For this review, take the finished solid that the model builds, in its own axes (mm). Face numbers are marked on the shaded views. Give positions to 0.01 mm unless a question says otherwise; leave off trailing zeros. Order: outer loops, then holes, each group sorted by start corner. A loop starts at its lowest first (then second) coordinate and runs counter-clockwise, first axis right, second up.
Item 1: Consider section D-D (z = -3). Give the boundary of the cut face in (x, y), plus the area to 3 significant figures.
Item 2: Consider section C-C (y = 0.25). Give the number of separate pieces and of enclosed holes in the cut face, plus the area to 3 significant figures.
Item 3: Consider section B-B (y = 2). Give the boundary of the cut face in (x, z), plus the area to 3 significant figures.
Item 4: For probe 1 along Z at (x, y) = (-0.5, 2.7); probe 2 along Y at (x, z) = (0, -4.25), list the stretches that pass through material, from the lowest coordinate up.
Item 5: Consider section A-A (x = 0). Give the boundary of the cut face in (y, z).
Item 6: The part is to be moulded in two halves that separate along Z. For the marked faces 1, 2 and 3, say which applies: released by +Z, released by -Z, zero draft, split by the parting line, or undercut.
Item 7: For P1, Ø1, axis at x = 11, y = -2.5, coming from the +Z side; P2, Ø1.6, axis at x = 9, y = 0.5, coming from the +Z side; P3, Ø0.6, axis at x = 8, z = -1, coming from the +Y side; P4, Ø6, axis at x = 7.5, z = -1.5, coming from the -Y side, all flat-tipped, find the tip position at first contact; note any pin that passes through.
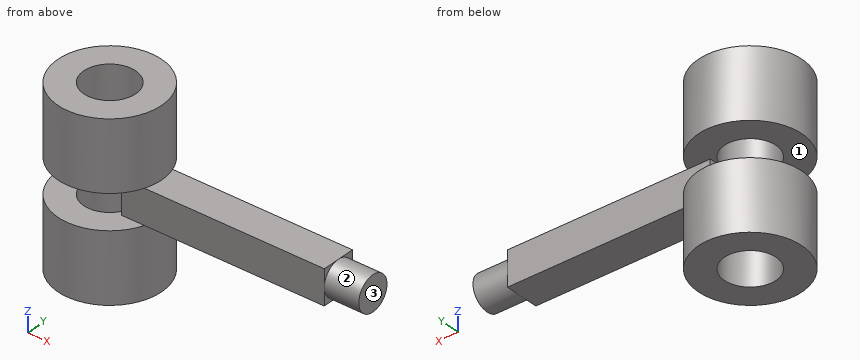
```python
from build123d import *

# Parameters (mm, degrees)
SKETCH1_R           = 3
SKETCH1_R_2         = 1.5
BOSS_EXTRUDE1_DEPTH = 4
SKETCH2_R           = 3
SKETCH2_R_2         = 1.5
BOSS_EXTRUDE2_DEPTH = 4
BOSS_EXTRUDE3_REACH = 9.348
SKETCH3_W           = 1
SKETCH3_H           = 2
SKETCH4_W           = 2
SKETCH4_H           = 2
BOSS_EXTRUDE4_DEPTH = 10.75
SKETCH6_R           = 1
BOSS_EXTRUDE5_DEPTH = 2


with BuildPart() as part:
    # Sketch1 → Boss-Extrude1 (new body)
    with BuildSketch(Plane.XY):
        Circle(SKETCH1_R)
        Circle(SKETCH1_R_2, mode=Mode.SUBTRACT)
    extrude(amount=BOSS_EXTRUDE1_DEPTH)

    # Sketch3 → Boss-Extrude3 (add, up to next)
    with BuildSketch(Plane.XY.offset(-2), mode=Mode.PRIVATE) as boss_extrude3_sk1:
        with Locations((2, 0)):
            Rectangle(SKETCH3_W, SKETCH3_H)
    boss_extrude3_tool1 = extrude(boss_extrude3_sk1.sketch, amount=BOSS_EXTRUDE3_REACH, mode=Mode.PRIVATE) - part.part


with BuildPart() as body_2:
    # Sketch2 → Boss-Extrude2 (new body)
    with BuildSketch(Plane(origin=(0, 0, -2), x_dir=(-1, 0, 0), z_dir=(0, 0, -1))):
        with Locations(Location((0, 0, 0), (0, 0, 180))):
            Circle(SKETCH2_R)
        with Locations(Location((0, 0, 0), (0, 0, 180))):
            Circle(SKETCH2_R_2, mode=Mode.SUBTRACT)
    extrude(amount=BOSS_EXTRUDE2_DEPTH)


with BuildPart() as part_1:
    add(part.part)

    add(body_2.part)  # Boss-Extrude3 merges body 2
    add(boss_extrude3_tool1.solids().sort_by_distance((2, 0, -2))[0])

    # Sketch4 → Boss-Extrude4 (add)
    with BuildSketch(Plane(origin=(2.5, 0, 0), x_dir=(0, 0, -1), z_dir=(1, 0, 0))):
        with Locations((1, 0)):
            Rectangle(SKETCH4_W, SKETCH4_H)
    extrude(amount=BOSS_EXTRUDE4_DEPTH)

    # Sketch6 → Boss-Extrude5 (add)
    with BuildSketch(Plane(origin=(13.25, 0, 0), x_dir=(0, 0, -1), z_dir=(1, 0, 0))):
        with Locations((1, 0)):
            Circle(SKETCH6_R)
    extrude(amount=BOSS_EXTRUDE5_DEPTH)


solid = part_1.part
```
Resolved:
1. outline: circle Ø6 at (0, 0); hole circle Ø3 at (0, 0)
1. area: 21.2 mm2
2. separate pieces: 3
2. enclosed holes: 0
2. area: 51.5 mm2
3. outline: (-2.24, -6) - (2.24, -6) - (2.24, -2) - (-2.24, -2) - close; (-2.24, 0) - (2.24, 0) - (2.24, 4) - (-2.24, 4) - close
3. area: 35.8 mm2
4. probe 1: z = -6 to -2, 0 to 4
4. probe 2: y = -3 to -1.5, 1.5 to 3
5. outline: (-3, -6) - (-1.5, -6) - (-1.5, -2) - (-3, -2) - close; (-3, 0) - (-1.5, 0) - (-1.5, 4) - (-3, 4) - close; (1.5, -6) - (3, -6) - (3, -2) - (1.5, -2) - close; (1.5, 0) - (3, 0) - (3, 4) - (1.5, 4) - close
6. face 1: undercut
6. face 2: split by the parting line
6. face 3: zero draft
7. P1: passes through
7. P2: stops at z = 0
7. P3: stops at y = 1
7. P4: stops at y = -1
